```python
from build123d import *

# Parameters (mm, degrees)
SKETCH1_R           = 3.175
BOSS_EXTRUDE1_DEPTH = 25.4
CUT_EXTRUDE1_START  = 50.8
SKETCH2_W           = 64.994311014
SKETCH2_H           = 38.1
CUT_EXTRUDE1_DEPTH  = 44.45
SKETCH3_R           = 4.7625
CUT_EXTRUDE2_DEPTH  = 65.240638337


with BuildPart() as part:
    # Sketch1 → Boss-Extrude1 (new, symmetric)
    with BuildSketch(Plane.XY):
        with BuildLine():
            Line((0, 0), (-9.376460946, 9.101647163))
            ThreePointArc((-9.376460946, 9.101647163), (-10.10301176, 31.130324977), (11.88494229, 32.653610572))
            Line((11.88494229, 32.653610572), (50.8, 0))
            Line((50.8, 0), (0, 0))
        make_face()
        with Locations((1.680688986, 20.492655038)):
            Circle(SKETCH1_R, mode=Mode.SUBTRACT)
    extrude(amount=BOSS_EXTRUDE1_DEPTH, both=True)

    # Sketch2 → Cut-Extrude1 (cut)
    with BuildSketch(Plane(origin=(0, 0, 0), x_dir=(1, 0, 0), z_dir=(0, 1, 0)).offset(CUT_EXTRUDE1_START)):
        with Locations((18.302844493, 0)):
            Rectangle(SKETCH2_W, SKETCH2_H)
    extrude(amount=-CUT_EXTRUDE1_DEPTH, mode=Mode.SUBTRACT)

    # Sketch3 → Cut-Extrude2 (cut, through all)
    with BuildSketch(Plane(origin=(0, 6.35, 0), x_dir=(1, 0, 0), z_dir=(0, 1, 0))):
        with Locations(Location((31.75, 0, 0), (0, 0, 270))):
            Circle(SKETCH3_R)
    extrude(amount=-CUT_EXTRUDE2_DEPTH, mode=Mode.SUBTRACT)


solid = part.part
```
Design review of the part built by this model. Coordinates are the model's own, in mm. A direction names the side the tool comes from. Coordinates: 2 decimals unless noted, no trailing zeros. Loops run counter-clockwise (first coordinate to the right, second up) from the corner with the lowest first, then second, coordinate; pieces in that order, holes last. Notation, with made-up numbers: M 17,-18.75 L 72,-18.75 A35 ccw 72,15.25 Z; hole C -26.5,80 d8. An arc over 180 degrees is marked long. One line per question, with ' | ' between items.
(1) Wall thickness on probe 1 along Z at (x, y) = (-8, 15.5); probe 2 along Y at (x, z) = (32, 7.5): over which ranges is each line inside the solid? List them lowest first.
Filled in:
probe 1: z = -25.4 to -19.05, 19.05 to 25.4 | probe 2: y = 0 to 6.35
(2) We need section B-B (x = 4). Give the boundary of the cut face in (y, z).
Filled in:
outline: M 0,-25.4 L 18.32,-25.4 L 18.32,-19.05 L 6.35,-19.05 L 6.35,19.05 L 18.32,19.05 L 18.32,25.4 L 0,25.4 Z; M 22.66,-25.4 L 36.2,-25.4 L 36.2,-19.05 L 22.66,-19.05 Z; M 22.66,19.05 L 36.2,19.05 L 36.2,25.4 L 22.66,25.4 Z
(3) We need section C-C (y = 8). Give the boundary of the cut face in (x, z).
Filled in:
outline: M -8.24,-25.4 L 41.27,-25.4 L 41.27,-19.05 L -8.24,-19.05 Z; M -8.24,19.05 L 41.27,19.05 L 41.27,25.4 L -8.24,25.4 Z
(4) We need section D-D (x = 33.5). Give the boundary of the cut face in (y, z), and give its area (3 significant figures).
Filled in:
outline: M 0,-25.4 L 14.52,-25.4 L 14.52,-19.05 L 6.35,-19.05 L 6.35,-4.43 L 0,-4.43 Z; M 0,4.43 L 6.35,4.43 L 6.35,19.05 L 14.52,19.05 L 14.52,25.4 L 0,25.4 Z | area: 370 mm^2
(5) Draft analysis for pull direction X (two halves, no side actions). For faces 3 (the face through (8, 18, -19.05)), 4 (the face through (-3.581, 3.476, 0.356)), 5 (the face through (-10.329, 30.875, 22.269)), 6 (the face through (0.992, 17.393, -22.269)), state which applies: released by +X, released by -X, zero draft, split by the parting line, or undercut.
Filled in:
face 3: zero draft | face 4: released by -X | face 5: split by the parting line | face 6: undercut
(6) We need section A-A (z = 0). Give the boundary of the cut face in (x, y), and give its area (3 significant figures).
Filled in:
outline: M -6.54,6.35 L 0,0 L 26.99,0 L 26.99,6.35 Z; M 36.51,0 L 50.8,0 L 43.23,6.35 L 36.51,6.35 Z | area: 259 mm^2
(7) For pin 1 Ø4 at (y, z) = (15, 19.5) entering from -X; pin 2 Ø5 at (y, z) = (7, -18) entering from +X, all flat-tipped, find the tip position at first contact; note any pin that passes through.
Filled in:
pin 1: stops at x = -13.81 | pin 2: stops at x = 45.44
(8) Machinability: for faces 1 (the face through (18, 6.35, 0)), 2 (the face through (36.47, 3.22, -0.62)), which of the approach directions +Z, -Z, +X, -X, +Y, -Y give a long, thin tool a straight path to every point of the face, cutting with its end or side? Answer none if there is none.
Filled in:
face 1: +X, -X, +Y | face 2: +Y, -Y
